from build123d import *

# Parameters (mm, degrees)
SKETCH3_W                = 152.4
SKETCH3_H                = 101.6
BOSS_EXTRUDE1_DEPTH      = 6.35
BOSS_EXTRUDE1_DEPTH_BACK = 6.35
FILLET1_R                = 0.4191
SKETCH5_R                = 3.4036
CUT_EXTRUDE2_DEPTH       = 13.7


with BuildPart() as part:
    # Sketch3 → Boss-Extrude1 (new body, two sides)
    with BuildSketch(Plane(origin=(0, 0, 0), x_dir=(1, 0, 0), z_dir=(0, 1, 0))) as boss_extrude1_sk:
        Rectangle(SKETCH3_W, SKETCH3_H)
    extrude(amount=BOSS_EXTRUDE1_DEPTH)
    extrude(boss_extrude1_sk.sketch, amount=-BOSS_EXTRUDE1_DEPTH_BACK)

    # Fillet1
    fillet1_edges = [part.edges().sort_by_distance(p)[0] for p in [
        (0, -6.35, -50.8),
        (0, -6.35, 50.8),
        (0, 6.35, -50.8),
        (0, 6.35, 50.8),
    ]]
    fillet(fillet1_edges, radius=FILLET1_R)

    # Sketch5 → Cut-Extrude2 (cut, through all)
    with BuildSketch(Plane(origin=(0, 6.35, 0), x_dir=(1, 0, 0), z_dir=(0, 1, 0))):
        with Locations((31.75, 31.75)):
            Circle(SKETCH5_R)
        with Locations((31.75, -31.75)):
            Circle(SKETCH5_R)
        with Locations((-31.75, -31.75)):
            Circle(SKETCH5_R)
        with Locations((-31.75, 31.75)):
            Circle(SKETCH5_R)
    extrude(amount=-CUT_EXTRUDE2_DEPTH, mode=Mode.SUBTRACT)


solid = part.part
CAD build for the part. Positions are in the model's coordinates, mm. Give positions to 0.01 mm unless a question says otherwise; leave off trailing zeros. Loops run counter-clockwise (first coordinate to the right, second up) from the corner with the lowest first, then second, coordinate; pieces in that order, holes last. Notation, with made-up numbers: M -31.75,0 L 12.25,0 A24 cw 12.25,11 Z; hole C 20.25,-0.5 d8. An arc over 180 degrees is marked long. Answer in a Markdown table with one row per item. Add a question column.
Item 1: Mould opens along Z. For faces 1 (the face through (-1, 0, -50.8)), 2 (the face through (-1, 6.35, -1)), 3 (the face through (29.24, 0.09, -34.05)), 4 (the face through (-34.26, 0.09, -34.05)) say: +Z half, -Z half, draft (parallel to the pull), parting line (faces both ways), or undercut.
Item 2: Probe probe 1 along Z at (x, y) = (31.75, -2.5); probe 2 along X at (y, z) = (0, -31.75). List the from-to ranges inside material, lowest first.
Item 3: Drop a flat-ended pin along its axis: P1, Ø4, axis at x = 31.75, z = 31.75, coming from the -Y side. Give the stop position or say it passes through.
Item 4: Band-saw the part on A-A on z = 31.75. Give the cut face in (x, y).
Item 5: Band-saw the part on B-B on x = -31.75. Give the cut face in (y, z).
Reply:
| question | item | result |
|---|---|---|
| 1 | face 1 | -Z half |
| 1 | face 2 | draft |
| 1 | face 3 | undercut |
| 1 | face 4 | undercut |
| 2 | probe 1 | z = -50.8 to -35.15, -28.35 to 28.35, 35.15 to 50.8 |
| 2 | probe 2 | x = -76.2 to -35.15, -28.35 to 28.35, 35.15 to 76.2 |
| 3 | P1 | passes through |
| 4 | outline | M -76.2,-6.35 L -35.15,-6.35 L -35.15,6.35 L -76.2,6.35 Z; M -28.35,-6.35 L 28.35,-6.35 L 28.35,6.35 L -28.35,6.35 Z; M 35.15,-6.35 L 76.2,-6.35 L 76.2,6.35 L 35.15,6.35 Z |
| 5 | outline | M -6.35,-50.38 A0.42 ccw -5.93,-50.8 L 5.93,-50.8 A0.42 ccw 6.35,-50.38 L 6.35,-35.15 L -6.35,-35.15 Z; M -6.35,-28.35 L 6.35,-28.35 L 6.35,28.35 L -6.35,28.35 Z; M -6.35,35.15 L 6.35,35.15 L 6.35,50.38 A0.42 ccw 5.93,50.8 L -5.93,50.8 A0.42 ccw -6.35,50.38 Z |
